Input: dimensioned drawing with shaded views. Units: mm. Origin: part minimum x, y, z. Coordinates: 2 decimals unless noted, no trailing zeros. Order: outer loops, then holes, each group sorted by start corner. A loop starts at its lowest first (then second) coordinate and runs counter-clockwise, first axis right, second up. Notation, with made-up numbers: (9.5, 29.5) -> (21.5, 29.5) arc R6 ccw to (21.5, 34.5) -> close; hole circle Ø3 at (15, -4). An arc over 180 degrees is marked (long way). Put each result on its own line as item: value.
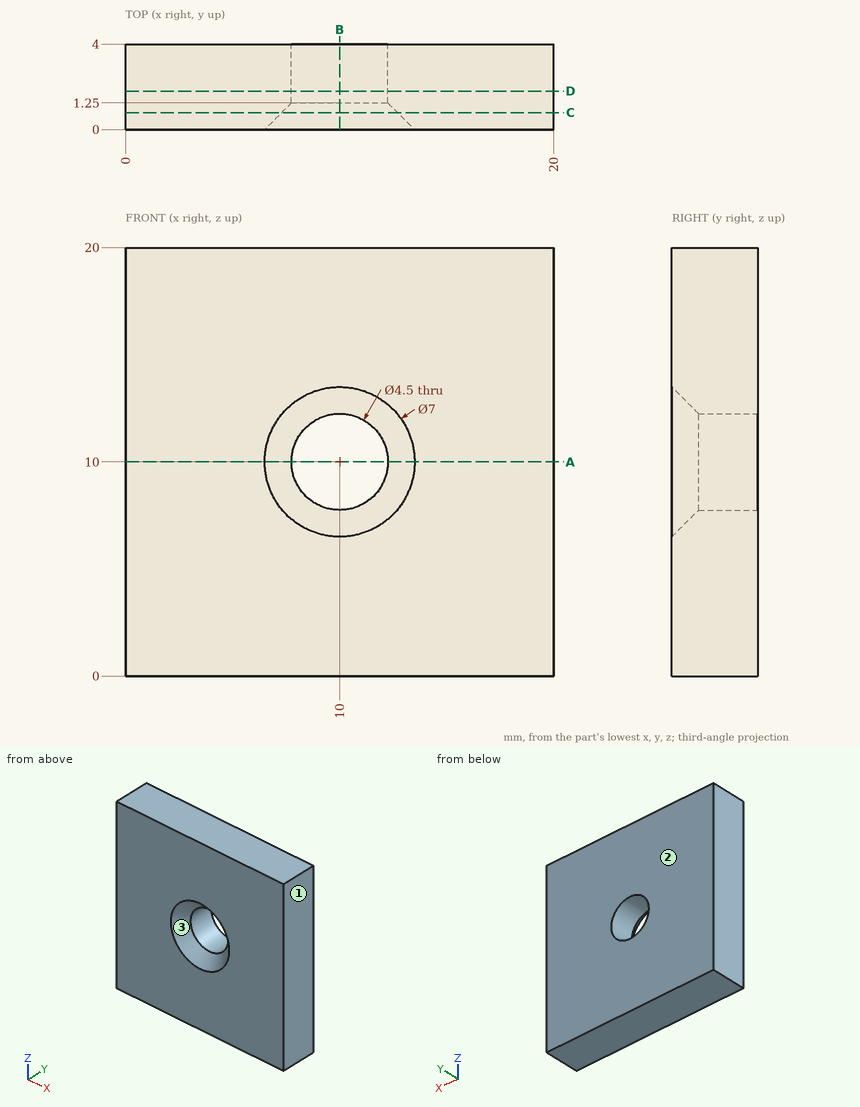
1. Ray query, line 1 along X through (y, z) = (2.05, 10); line 2 along Z through (x, y) = (10.75, 0.9). Return the intervals inside material, ascending.
Numbers:
line 1: x = 0 to 7.75, 12.25 to 20
line 2: z = 0 to 7.51, 12.49 to 20
2. Cut plane A-A on z = 10. Output: boundary loops of the cut face in (x, y), plus the area to 3 significant figures.
Numbers:
outline: (0, 0) -> (6.5, 0) -> (7.75, 1.25) -> (7.75, 4) -> (0, 4) -> close; (12.25, 1.25) -> (13.5, 0) -> (20, 0) -> (20, 4) -> (12.25, 4) -> close
area: 60.4 mm2
3. Pull-direction query (X, two-part tool) for the marked faces 1, 2 and 3; classes: pulls with the +X half, pulls with the -X half, needs draft (parallel to the pull), parting line crosses it, or undercut.
Numbers:
face 1: pulls with the +X half
face 2: needs draft
face 3: undercut
4. Cut plane C-C on y = 0.8. Output: boundary loops of the cut face in (x, z), plus the area to 3 significant figures.
Numbers:
outline: (0, 0) -> (20, 0) -> (20, 20) -> (0, 20) -> close; hole circle Ø5.4 at (10, 10)
area: 377 mm2
5. Cut plane D-D on y = 1.8. Output: boundary loops of the cut face in (x, z).
Numbers:
outline: (0, 0) -> (20, 0) -> (20, 20) -> (0, 20) -> close; hole circle Ø4.5 at (10, 10)
6. Cut plane B-B on x = 10. Output: boundary loops of the cut face in (y, z).
Numbers:
outline: (0, 0) -> (4, 0) -> (4, 7.75) -> (1.25, 7.75) -> (0, 6.5) -> close; (0, 13.5) -> (1.25, 12.25) -> (4, 12.25) -> (4, 20) -> (0, 20) -> close
